Can you work these out from the model? Positions are in its coordinate system, mm. Face numbers are marked on the shaded views. A direction names the side the tool comes from. Coordinates: 2 decimals unless noted, no trailing zeros. Order: outer loops, then holes, each group sorted by start corner. A loop starts at its lowest first (then second) coordinate and runs counter-clockwise, first axis right, second up. Notation, with made-up numbers: (-20.5, 49.25) -> (-4.5, 49.25) arc R23 cw to (-4.5, 69.25) -> close; hole circle Ø6 at (69, 77.25). An arc over 180 degrees is marked (long way). Write item = value, one per line.
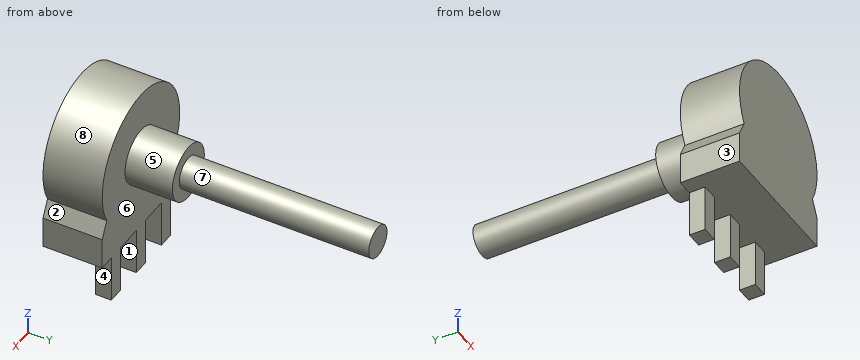
```python
from build123d import *

# Parameters (mm, degrees)
F1_DEPTH = 7.5
F0_W     = 2
F0_H     = 6
F2_DEPTH = 2
F3_R     = 3.5
F4_DEPTH = 6
F5_R     = 2
F6_DEPTH = 24


with BuildPart() as f1:
    # F0 (on Front) → F1 (new body)
    with BuildSketch(Plane.XZ):
        with BuildLine():
            Line((-7.5, -4), (7.5, -4))
            ThreePointArc((7.5, -4), (0, 8.5), (-7.5, -4))
        make_face()
        Polygon((8.5, -6), (7.5, -4), (-7.5, -4), (-8.5, -6), (-8.5, -10), (-6.5, -10), (-4.5, -10), (-1, -10), (0, -10), (1, -10), (4.5, -10), (6.5, -10), (8.5, -10), align=None)
    extrude(amount=F1_DEPTH)

    # F0 (on Front) → F2 (join)
    with BuildSketch(Plane.XZ):
        with Locations((-5.5, -13)):
            Rectangle(F0_W, F0_H)
        Polygon((1, -16), (1, -10), (0, -10), (-1, -10), (-1, -16), align=None)
        with Locations((5.5, -13)):
            Rectangle(F0_W, F0_H)
    extrude(amount=F2_DEPTH)

    # F3 (on face) → F4 (join)
    with BuildSketch(Plane.XZ):
        Circle(F3_R)
    extrude(amount=-F4_DEPTH)

    # F5 (on face) → F6 (join)
    with BuildSketch(Plane(origin=(0, 6, 0), x_dir=(-1, 0, 0), z_dir=(0, 1, 0))):
        Circle(F5_R)
    extrude(amount=F6_DEPTH)


solid = f1.part
```
Item 1: I want a section at B-B, the plane x = 0. Please give me the cut outline in (y, z).
A:
outline = (-7.5, -10) -> (-2, -10) -> (-2, -16) -> (0, -16) -> (0, -3.5) -> (6, -3.5) -> (6, -2) -> (30, -2) -> (30, 2) -> (6, 2) -> (6, 3.5) -> (0, 3.5) -> (0, 8.5) -> (-7.5, 8.5) -> close
Item 2: I want a section at D-D, the plane z = -9.25. Please give me the cut outline in (x, y).
A:
outline = (-8.5, -7.5) -> (8.5, -7.5) -> (8.5, 0) -> (-8.5, 0) -> close
Item 3: If we mould it in two halves opening along Z, with no side actions, what happens to the marked faces 6, 7 and 8? For each: pulls with the +Z half, pulls with the -Z half, needs draft (parallel to the pull), parting line crosses it, or undercut.
A:
face_6 = needs draft
face_7 = parting line crosses it
face_8 = undercut
Item 4: I want a section at C-C, the plane y = 13. Please give me the cut outline in (x, z), plus the area to 3 significant figures.
A:
outline = circle Ø4 at (0, 0)
area = 12.6 mm2
Item 5: If I drill on probe 1 along Y at (x, z) = (-2.75, 7.75); probe 2 along Y at (x, z) = (-2, -1.5); probe 3 along Z at (x, y) = (4.25, -4.5), over which ranges is the centre line in solid material (lowest first)?
A:
probe_1 = -7.5 to 0
probe_2 = -7.5 to 6
probe_3 = -10 to 7.36
Item 6: For the marked faces 1, 2, 3, 4 and 5, which set-ups out of +Z, -Z, +X, -X, +Y, -Y let a thin tool reach every point of the face, with its end or its side?
A:
face_1 = -Z, +Y, -Y
face_2 = +X, +Y, -Y
face_3 = +Z, -Z, -X, +Y, -Y
face_4 = -Z, +X, +Y, -Y
face_5 = +Y
Item 7: I'm going to push flat-ended pins straight in: P1, Ø1, axis at x = -5, z = -12.5, coming from the -Y side; P2, Ø1, axis at y = -1.5, z = -12, coming from the -X side; P3, Ø2, axis at y = -0.5, z = -12.5, coming from the +X side. Where does each tip first touch, or does it pass through?
A:
P1 = -2
P2 = -6.5
P3 = 6.5
Item 8: I want a section at A-A, the plane z = 0. Please give me the cut outline in (x, y).
A:
outline = (-8.5, -7.5) -> (8.5, -7.5) -> (8.5, 0) -> (3.5, 0) -> (3.5, 6) -> (2, 6) -> (2, 30) -> (-2, 30) -> (-2, 6) -> (-3.5, 6) -> (-3.5, 0) -> (-8.5, 0) -> close
